Read the model definition and answer for the solid it produces. Units are mm, in the model's axes. A direction names the side the tool comes from. Coordinates: 2 decimals unless noted, no trailing zeros. Loops run counter-clockwise (first coordinate to the right, second up) from the corner with the lowest first, then second, coordinate; pieces in that order, holes last. Notation, with made-up numbers: (54.25, -20) -> (80.25, -20) arc R7 ccw to (80.25, -14) -> close; hole circle Ø7 at (28.25, 72.5). An arc over 180 degrees is marked (long way). Answer as a JSON object with one key per item and string values. Group by question number.
Q1. The part is cut by section C-C on x = 0. Write down the section's boundary in (y, z), and give its area (3 significant figures).
Q2. The part is cut by section D-D on y = 6.75. Write down the section's boundary in (x, z), and give its area (3 significant figures).
Q3. Straight lines are drawn through the part: line 1 along Y through (x, z) = (0, 27); line 2 along Z through (x, y) = (-1.5, 4); line 3 along X through (y, z) = (1.5, 33). For each, find the intervals that lie inside material, in ascending order. Write a range as [from, to].
Q4. Determine the mould class of faces 5 (the flat face through (0, -8, 50)), 6 (the flat face through (0, -10, -5)), 7 (the flat face through (0, 0, 0)) for opening direction Y: released by +Y, released by -Y, zero draft, split by the parting line, or undercut.
Q5. The part is cut by section B-B on z = 27. Write down the section's boundary in (x, y), and give its area (3 significant figures).
Q6. Each of these flat-tipped pins is pushed along its axis until it touches: P1, Ø1.5, axis at x = 0, z = 27, coming from the -Y side; P2, Ø3, axis at y = -0.5, z = -3.5, coming from the -X side; P3, Ø10, axis at y = 6, z = 19, coming from the -X side. Where does it stop, or does it pass through?
Q7. The part is cut by section A-A on y = -5.5. Write down the section's boundary in (x, z), and give its area (3 significant figures).
Q8. For faces 1 (the flat face through (0, -6, 48.7)), 2 (the flat face through (1.1, -6, 47)), 3 (the flat face through (-1.1, -6, 47)), 4 (the cylindrical face through (0, -2, 25)), determine the directions among +Z, -Z, +X, -X, +Y, -Y from which every point of the face is accessible in a straight line to the end or side of a thin tool.
from build123d import *

# Parameters (mm, degrees)
F0_R          = 3.5
F0_R_2        = 2
F1_DEPTH      = 50
F2_W          = 2.2
F2_H          = 5.43
F3_DEPTH      = 9.02
F4_END_RADIUS = 2
F4_REACH      = 14.8797455995
F5_W          = 2.2
F5_H          = 1.6
F6_DEPTH      = 1.3
F7_W          = 6
F7_H          = 20
F8_DEPTH      = 10


with BuildPart() as f1:
    # F0 (on Top) → F1 (new body)
    with BuildSketch(Plane.XY):
        Circle(F0_R)
        Circle(F0_R_2, mode=Mode.SUBTRACT)
    extrude(amount=F1_DEPTH)

    # F2 (on Front) → F3 (join)
    with BuildSketch(Plane.XZ):
        with Locations((0, 47.285)):
            Rectangle(F2_W, F2_H)
    extrude(amount=F3_DEPTH)

    f4_end = (Plane(origin=(0, 0, 25), x_dir=(-1, 0, 0), z_dir=(0, 0, -1)) * Cylinder(F4_END_RADIUS, 133.7931472917, mode=Mode.PRIVATE)).faces().sort_by_distance((-2, 0, 25))[0]
    # F2 (on Front) → F4 (cut, up to the whole of a round face its end follows)
    with BuildSketch(Plane.XZ):
        with Locations((0, 47.285)):
            Rectangle(F2_W, F2_H)
    f4_long = extrude(amount=F4_REACH, mode=Mode.PRIVATE)
    add(split(f4_long, bisect_by=f4_end, keep=Keep.BOTTOM, mode=Mode.PRIVATE), mode=Mode.SUBTRACT)

    # F5 (on face) → F6 (cut)
    with BuildSketch(Plane.XY.offset(50)):
        with Locations((0, -5.57)):
            Rectangle(F5_W, F5_H)
    extrude(amount=-F6_DEPTH, mode=Mode.SUBTRACT)

    # F7 (on face) → F8 (join)
    with BuildSketch(Plane(origin=(0, 0, 0), x_dir=(1, 0, 0), z_dir=(0, 0, -1))):
        Rectangle(F7_W, F7_H)
    extrude(amount=F8_DEPTH)


solid = f1.part
Final values:
{
 "1": {"outline": "(-10, -10) -> (10, -10) -> (10, 0) -> (3.5, 0) -> (3.5, 50) -> (2, 50) -> (2, 0) -> (-2, 0) -> (-2, 50) -> (-4.77, 50) -> (-4.77, 48.7) -> (-6.37, 48.7) -> (-6.37, 50) -> (-9.02, 50) -> (-9.02, 44.57) -> (-3.5, 44.57) -> (-3.5, 0) -> (-10, 0) -> close", "area": "378 mm2"},
 "2": {"outline": "(-3, -10) -> (3, -10) -> (3, 0) -> (-3, 0) -> close", "area": "60.0 mm2"},
 "3": {"line 1": "y = [-3.5, -2], [2, 3.5]", "line 2": "z = [-10, 0]", "line 3": "x = [-3.16, -1.32], [1.32, 3.16]"},
 "4": {"face 5": "zero draft", "face 6": "released by -Y", "face 7": "undercut"},
 "5": {"outline": "circle Ø7 at (0, 0); hole circle Ø4 at (0, 0)", "area": "25.9 mm2"},
 "6": {"P1": "stops at y = -3.5", "P2": "stops at x = -3", "P3": "stops at x = -3.35"},
 "7": {"outline": "(-3, -10) -> (3, -10) -> (3, 0) -> (-3, 0) -> close; (-1.1, 44.57) -> (1.1, 44.57) -> (1.1, 48.7) -> (-1.1, 48.7) -> close", "area": "69.1 mm2"},
 "8": {"face 1": "+Z, +X, -X", "face 2": "+Z, +X, -Y", "face 3": "+Z, -X, -Y", "face 4": "+Z"}
}
